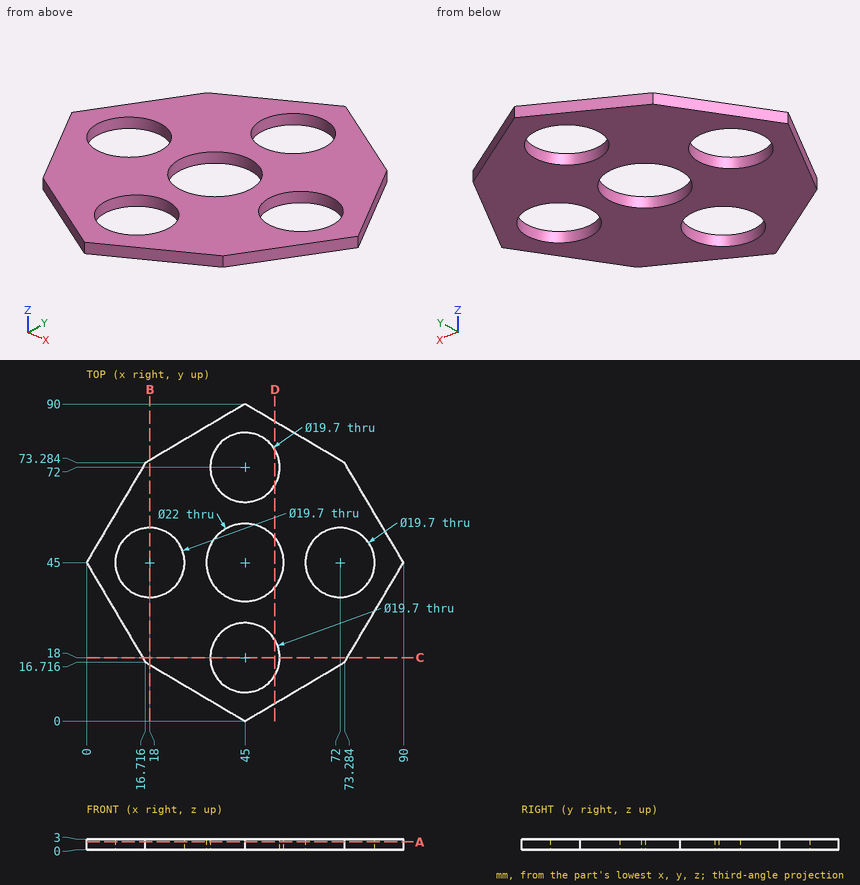
Print and shaded views of the part. All mm, measured from the part's lowest x, y and z. Give positions to 0.01 mm unless a question says otherwise; leave off trailing zeros. Order: outer loops, then holes, each group sorted by start corner. A loop starts at its lowest first (then second) coordinate and runs counter-clockwise, first axis right, second up. Notation, with made-up numbers: (23.25, -37) -> (36.25, -37) arc R29 cw to (36.25, -8) -> close; hole circle Ø5 at (-17.5, 23). An arc over 180 degrees is marked (long way). Use CSV: the item, a comma, the result in double quotes.
1. Drop flat-ended pins along their axis: pin 1 (12 mm diameter, centred on x = 18, y = 45, fed in from +Z); pin 2 (1.5 mm diameter, centred on y = 43, z = 2, fed in from +X). Give the stop position or say it passes through.
Outcome:
pin 1,"through"
pin 2,"x = 89.26"
2. Band-saw the part on A-A, the plane z = 2.2. Give the cut face in (x, y), then the cut area to 3 significant figures.
Outcome:
outline,"(0, 45) -> (16.72, 16.72) -> (45, 0) -> (73.28, 16.72) -> (90, 45) -> (73.28, 73.28) -> (45, 90) -> (16.72, 73.28) -> close; hole circle Ø19.7 at (18, 45); hole circle Ø22 at (45, 45); hole circle Ø19.7 at (45, 18); hole circle Ø19.7 at (45, 72); hole circle Ø19.7 at (72, 45)"
area,"3,490 mm²"
3. Drill centre lines: line 1 along Y through (x, z) = (45, 2); line 2 along Y through (x, z) = (13, 2.5) (1 decimal); line 3 along X through (y, z) = (64.5, 2.6) (1 decimal). Where is each one in solid material? Low to high. Write a range as from..to.
Outcome:
line 1,"0..8.15, 27.85..34, 56..62.15, 81.85..90"
line 2,"23..36.5, 53.5..67"
line 3,"11.5..38.6, 51.4..78.5"
4. Band-saw the part on D-D, the plane x = 53.5. Give the cut face in (y, z).
Outcome:
outline,"(5.02, 0) -> (13.02, 0) -> (13.02, 3) -> (5.02, 3) -> close; (22.98, 0) -> (38.02, 0) -> (38.02, 3) -> (22.98, 3) -> close; (51.98, 0) -> (67.02, 0) -> (67.02, 3) -> (51.98, 3) -> close; (76.98, 0) -> (84.98, 0) -> (84.98, 3) -> (76.98, 3) -> close"
5. Band-saw the part on B-B, the plane x = 18. Give the cut face in (y, z).
Outcome:
outline,"(15.96, 0) -> (35.15, 0) -> (35.15, 3) -> (15.96, 3) -> close; (54.85, 0) -> (74.04, 0) -> (74.04, 3) -> (54.85, 3) -> close"
